Geometry: final body of the model. Coordinates: model frame, mm. A direction names the side the tool comes from. Round coordinates to 2 decimals unless told otherwise and drop trailing zeros. Loops run counter-clockwise (first coordinate to the right, second up) from the corner with the lowest first, then second, coordinate; pieces in that order, holes last. Notation, with made-up numbers: M 71,-12 L 97,-12 A23 cw 97,12 Z; hole C -39,4 d2. An arc over 180 degrees is marked long. Answer as a JSON object with one key per item and string values.
from build123d import *

# Parameters (mm, degrees)
SKETCH_1_W          = 90
SKETCH_1_H          = 75
EXTRUDE_1_DEPTH     = 5
SKETCH_3_W          = 40
SKETCH_3_H          = 3
EXTRUDE_2_DEPTH     = 20
SKETCH_4_R          = 2.65
CUT_EXTRUDE_2_DEPTH = 20
SKETCH_5_W          = 85
SKETCH_5_H          = 69
CUT_EXTRUDE_3_DEPTH = 3


with BuildPart() as part:
    # 草图1 → 凸台-拉伸1 (new body)
    with BuildSketch(Plane.XY):
        with Locations((-1.168582375, -16.58045977)):
            Rectangle(SKETCH_1_W, SKETCH_1_H)
    extrude(amount=EXTRUDE_1_DEPTH)

    # 草图3 → 凸台-拉伸2 (add)
    with BuildSketch(Plane(origin=(0, 0, 0), x_dir=(-1, 0, 0), z_dir=(0, 0, -1))):
        with Locations((1.168582375, 19.41954023)):
            Rectangle(SKETCH_3_W, SKETCH_3_H)
    extrude(amount=EXTRUDE_2_DEPTH)

    # 草图4 → 切除-拉伸2 (cut)
    with BuildSketch(Plane(origin=(0, 20.91954023, 0), x_dir=(1, 0, 0), z_dir=(0, 1, 0))):
        with Locations((-1.168582375, 10)):
            Circle(SKETCH_4_R)
    extrude(amount=-CUT_EXTRUDE_2_DEPTH, mode=Mode.SUBTRACT)

    # 草图5 → 切除-拉伸3 (cut)
    with BuildSketch(Plane(origin=(0, 0, 0), x_dir=(-1, 0, 0), z_dir=(0, 0, -1))):
        with Locations((1.475961606, -17.646255622)):
            Rectangle(SKETCH_5_W, SKETCH_5_H)
    extrude(amount=-CUT_EXTRUDE_3_DEPTH, mode=Mode.SUBTRACT)


solid = part.part
1) Pull-direction query (X, two-part tool) for faces 6 (the flat face through (-21.169, 19, -10)), 7 (the flat face through (-1, 16.854, 1)), 8 (the flat face through (-2, -54.08, 2)); classes: +X half, -X half, draft (parallel to the pull), parting line (faces both ways), or undercut.
Results:
{"face 6": "-X half", "face 7": "undercut", "face 8": "draft"}
2) Reachability of faces 1 (the flat face through (4, 17.92, -10)), 2 (the flat face through (18.831, 19, -10)), 3 (the flat face through (43.831, -17, 2)), 4 (the flat face through (-43.976, -18, 1)), 5 (the cylindrical face through (-1.743, 19.441, -7.413)) from +Z, -Z, +X, -X, +Y, -Y: full face, straight path, thin tool, end or side. Return the list, or none.
Results:
{"face 1": "-Z, +X, -X, -Y", "face 2": "-Z, +X, +Y, -Y", "face 3": "+Z, -Z, +X, +Y, -Y", "face 4": "-Z", "face 5": "+Y, -Y"}
3) Section query A-A (z = -10). Return the cut outline in (x, y), and give its area (3 significant figures).
Results:
{"outline": "M -21.17,17.92 L -3.82,17.92 L -3.82,20.92 L -21.17,20.92 Z; M 1.48,17.92 L 18.83,17.92 L 18.83,20.92 L 1.48,20.92 Z", "area": "104 mm2"}
4) Section query D-D (x = -16). Return the cut outline in (y, z).
Results:
{"outline": "M -54.08,0 L -52.15,0 L -52.15,3 L 16.85,3 L 16.85,0 L 17.92,0 L 17.92,-20 L 20.92,-20 L 20.92,5 L -54.08,5 Z"}
5) Section query B-B (y = -11.5). Return the cut outline in (x, z).
Results:
{"outline": "M -46.17,0 L -43.98,0 L -43.98,3 L 41.02,3 L 41.02,0 L 43.83,0 L 43.83,5 L -46.17,5 Z"}
6) Pin query (flat end, axial travel): P1, Ø8.5, axis at x = -1.17, z = -10, coming from the +Y side; P2, Ø0.9, axis at y = 19.5, z = -6, coming from the -X side; P3, Ø1, axis at x = -20.5, z = -15, coming from the -Y side; P4, Ø2.5, axis at y = 19, z = -10.5, coming from the +X side. Return the tip coordinate at first contact, or that it passes through.
Results:
{"P1": "y = 20.92", "P2": "x = -21.17", "P3": "y = 17.92", "P4": "x = 18.83"}
7) Ray query, line 1 (X direction, y = -17, z = 2); line 2 (X direction, y = 18.8, z = -10); line 3 (Y direction, x = -20.5, z = 1). Return the intervals inside material, ascending.
Results:
{"line 1": "-46.17 to -43.98, 41.02 to 43.83", "line 2": "-21.17 to -3.82, 1.48 to 18.83", "line 3": "-54.08 to -52.15, 16.85 to 20.92"}
8) Section query C-C (z = 2). Return the cut outline in (x, y), and give its area (3 significant figures).
Results:
{"outline": "M -46.17,-54.08 L 43.83,-54.08 L 43.83,20.92 L -46.17,20.92 Z; hole M -43.98,-52.15 L 41.02,-52.15 L 41.02,16.85 L -43.98,16.85 Z", "area": "885 mm2"}
